```python
from build123d import *

# Parameters (mm, degrees)
EXTRUDE_1_DEPTH     = 10
SKETCH_2_R          = 1.55
CUT_EXTRUDE_1_DEPTH = 26.946195882
SKETCH_3_R          = 2.5
CUT_EXTRUDE_2_DEPTH = 1.7
CUT_EXTRUDE_3_DEPTH = 26.946195882


with BuildPart() as part:
    # 스케치1 → 보스-돌출1 (new body)
    with BuildSketch(Plane.XY):
        Polygon((-10, 0), (0, 0), (0, 15), (-18.660254038, 15), align=None)
        with BuildLine():
            ThreePointArc((-10.232050808, 5.401923789), (-9.5, 8.133974596), (-6.767949192, 7.401923789))
            Line((-6.767949192, 7.401923789), (-4.767949192, 3.937822174))
            ThreePointArc((-4.767949192, 3.937822174), (-4.568148347, 3.455460264), (-4.5, 2.937822174))
            ThreePointArc((-4.5, 2.937822174), (-5.98236191, 1.005970521), (-8.232050808, 1.937822174))
            Line((-8.232050808, 1.937822174), (-10.232050808, 5.401923789))
        make_face(mode=Mode.SUBTRACT)
        with BuildLine():
            ThreePointArc((-8.5, 9.5), (-10.5, 11.5), (-8.5, 13.5))
            Line((-8.5, 13.5), (-6.5, 13.5))
            ThreePointArc((-6.5, 13.5), (-5.085786438, 12.914213562), (-4.5, 11.5))
            ThreePointArc((-4.5, 11.5), (-5.085786438, 10.085786438), (-6.5, 9.5))
            Line((-6.5, 9.5), (-8.5, 9.5))
        make_face(mode=Mode.SUBTRACT)
    extrude(amount=EXTRUDE_1_DEPTH)

    # 스케치2 → 컷-돌출1 (cut, through all)
    with BuildSketch(Plane.XZ):
        with Locations((0, 5)):
            Circle(SKETCH_2_R)
    extrude(amount=-CUT_EXTRUDE_1_DEPTH, mode=Mode.SUBTRACT)

    # 스케치3 → 컷-돌출2 (cut)
    with BuildSketch(Plane(origin=(0, 15, 0), x_dir=(1, 0, 0), z_dir=(0, 1, 0))):
        with Locations((0, -5)):
            Circle(SKETCH_3_R)
    extrude(amount=-CUT_EXTRUDE_2_DEPTH, mode=Mode.SUBTRACT)

    # 스케치4 → 컷-돌출3 (cut, through all)
    with BuildSketch(Plane.XY.offset(10)):
        Polygon((-18.660254038, 15), (-16.660254038, 15), (-16.660254038, 11.535898385), align=None)
    extrude(amount=-CUT_EXTRUDE_3_DEPTH, mode=Mode.SUBTRACT)


solid = part.part
```
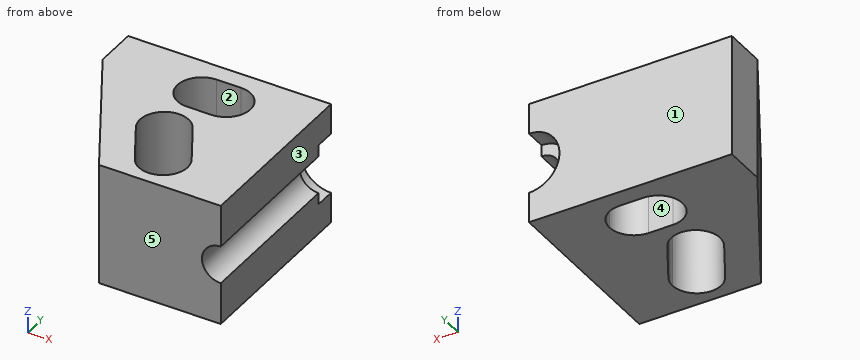
Here's how the part is built. I have some questions about the finished solid (model axes, mm). Face numbers are marked on the shaded views. A direction names the side the tool comes from. Give positions to 0.01 mm unless a question says otherwise; leave off trailing zeros. Order: outer loops, then holes, each group sorted by start corner. A loop starts at its lowest first (then second) coordinate and runs counter-clockwise, first axis right, second up. Notation, with made-up numbers: M 14,19.5 L 54,19.5 A27 ccw 54,42.5 Z; hole C 17,65.25 d3. An arc over 180 degrees is marked long. Use a Markdown table: item, result. Add a question column.
1. Suppose I cut it at D-D (z = 0.75). List the corners of the cut face in (x, y) for me, and give its area (3 significant figures).
2. I need wall thicknesses on probe 1 along Y at (x, z) = (-9, 6); probe 2 along Y at (x, z) = (-9.25, 2); probe 3 along Y at (x, z) = (-1.5, 3.75). Which ranges of each line are inside material? Lowest first, please. Write a range as from..to.
3. If we mould it in two halves opening along X, with no side actions, what happens to the marked faces 1, 2 and 3? For each: +X half, -X half, draft (parallel to the pull), parting line (faces both ways), or undercut.
4. On a 3-axis mill with a long thin cutter (end or side, diameter ignored), from which of +Z, -Z, +X, -X, +Y, -Y can I reach the whole of each face in a straight line? I mean the marked faces 4 and 5. Say none if no direction works.
5. Suppose I cut it at C-C (y = 13). List the corners of the cut face in (x, z) for me.
6. For pin 1 Ø3 at (x, z) = (-12, 3.5) entering from -Y; pin 2 Ø0.8 at (x, z) = (-1.5, 4) entering from +Y, each with a flat end and sliding along its axis, tell me the tip position at first contact or that it passes through.
7. Suppose I cut it at B-B (x = -6.25). List the corners of the cut face in (y, z) for me.
8. Suppose I cut it at A-A (z = 5). List the corners of the cut face in (x, y) for me, and give its area (3 significant figures).
Results list:
| question | item | result |
|---|---|---|
| 1 | outline | M -16.66,11.54 L -10,0 L 0,0 L 0,15 L -16.66,15 Z; hole M -10.23,5.4 L -8.23,1.94 A2 ccw -4.77,3.94 L -6.77,7.4 A2 ccw Z; hole M -8.5,9.5 L -6.5,9.5 A2 ccw -6.5,13.5 L -8.5,13.5 A2 ccw Z |
| 1 | area | 162 mm² |
| 2 | probe 1 | y = 0..3.27, 8.34..9.56, 13.44..15 |
| 2 | probe 2 | y = 0..3.7, 8.26..9.65, 13.35..15 |
| 2 | probe 3 | y = 0..13.3 |
| 3 | face 1 | draft |
| 3 | face 2 | undercut |
| 3 | face 3 | +X half |
| 4 | face 4 | +Z, -Z |
| 4 | face 5 | +Z, -Z, +X, -X, -Y |
| 5 | outline | M -16.66,0 L -9.82,0 L -9.82,10 L -16.66,10 Z; M -5.18,0 L 0,0 L 0,3.45 A1.55 cw 0,6.55 L 0,10 L -5.18,10 Z |
| 6 | pin 1 | stops at y = 0.87 |
| 6 | pin 2 | stops at y = 13.3 |
| 7 | outline | M 0,0 L 0.95,0 L 0.95,10 L 0,10 Z; M 6.5,0 L 9.52,0 L 9.52,10 L 6.5,10 Z; M 13.48,0 L 15,0 L 15,10 L 13.48,10 Z |
| 8 | outline | M -16.66,11.54 L -10,0 L -1.55,0 L -1.55,13.3 L -2.5,13.3 L -2.5,15 L -16.66,15 Z; hole M -10.23,5.4 L -8.23,1.94 A2 ccw -4.77,3.94 L -6.77,7.4 A2 ccw Z; hole M -8.5,9.5 L -6.5,9.5 A2 ccw -6.5,13.5 L -8.5,13.5 A2 ccw Z |
| 8 | area | 137 mm² |
